Input: part model. Units: mm. Frame: model coordinates. Face numbers are marked on the shaded views. A direction names the side the tool comes from. Give positions to 0.01 mm unless a question says otherwise; leave off trailing zeros. Write each loop counter-clockwise with the first axis right and the second up, starting at its lowest first coordinate (ties: lowest second). Pieces come first, ordered by that corner, then holes. Notation, with made-up numbers: (-25, 60) - (27, 60) arc R31 cw to (27, 90) - close; hole circle Ø5 at (53.5, -8). An arc over 180 degrees is marked (long way). Answer as a JSON object with one key per item and string values. Group by question number.
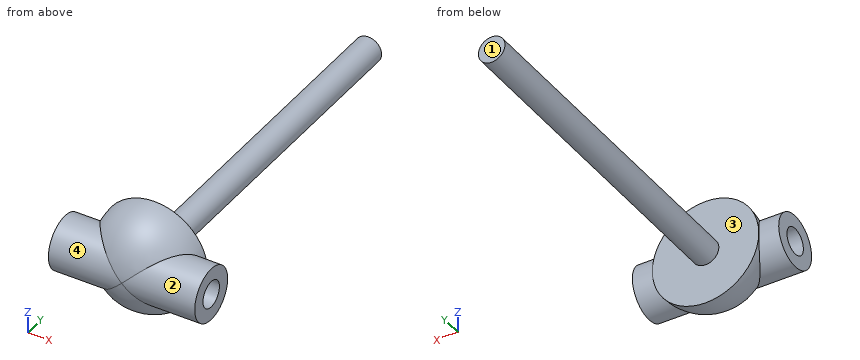
from build123d import *

# Parameters (mm, degrees)
OBR_T1_ANGLE                     = 180
DODANIE_WYCI_GNI_CIE1_DEPTH      = 27.5
DODANIE_WYCI_GNI_CIE1_DEPTH_BACK = 27.5
SZKIC4_R                         = 10
SZKIC5_R                         = 5
WYTNIJ_WYCI_GNI_CIE1_DEPTH       = 62.846584506
SZKIC6_R                         = 5
DODANIE_WYCI_GNI_CIE2_DEPTH      = 130


with BuildPart() as part:
    # Szkic3 → Obr_t1 (revolve)
    with BuildSketch(Plane(origin=(0, 0, 0), x_dir=(1, 0, 0), z_dir=(0, 1, 0))):
        with BuildLine():
            Line((0, 20), (0, -20))
            ThreePointArc((0, -20), (20, 0), (0, 20))
        make_face()
    revolve(axis=Axis((0, 0, -20), (0, 0, -1)), revolution_arc=OBR_T1_ANGLE)

    # Szkic4 → Dodanie-wyci_gni_cie1 (add, two sides: drawn at the far end of the back side and taken through both)
    with BuildSketch(Plane(origin=(0, 0, 0), x_dir=(0, 0, -1), z_dir=(1, 0, 0)).offset(-DODANIE_WYCI_GNI_CIE1_DEPTH_BACK)):
        with Locations((0, -10)):
            Circle(SZKIC4_R)
    extrude(amount=DODANIE_WYCI_GNI_CIE1_DEPTH + DODANIE_WYCI_GNI_CIE1_DEPTH_BACK)

    # Szkic5 → Wytnij-wyci_gni_cie1 (cut, through all)
    with BuildSketch(Plane(origin=(27.5, 0, 0), x_dir=(0, 0, -1), z_dir=(1, 0, 0))):
        with Locations((0, -10)):
            Circle(SZKIC5_R)
    extrude(amount=-WYTNIJ_WYCI_GNI_CIE1_DEPTH, mode=Mode.SUBTRACT)

    # Szkic6 → Dodanie-wyci_gni_cie2 (add)
    with BuildSketch(Plane(origin=(0, 0, 0), x_dir=(1, 0, 0), z_dir=(0, 1, 0))):
        with Locations(Location((0, 0, 0), (0, 0, 180))):
            Circle(SZKIC6_R)
    extrude(amount=DODANIE_WYCI_GNI_CIE2_DEPTH)


solid = part.part
1) Reachability of the marked faces 1, 2, 3 and 4 from +Z, -Z, +X, -X, +Y, -Y: full face, straight path, thin tool, end or side. Return the list, or none.
2) Pin query (flat end, axial travel): P1, Ø4, axis at x = 14, z = 7.5, coming from the +Y side; P2, Ø2, axis at y = 44, z = 1, coming from the +X side; P3, Ø12, axis at x = -3, y = 111, coming from the +Z side. Return the tip coordinate at first contact, or that it passes through.
3) Cut plane D-D on y = 24.5. Return the cut outline in (x, z).
4) Cut plane B-B on y = -10. Return the cut outline in (x, z), and give its area (3 significant figures).
5) Line query: line 1 along Y through (x, z) = (7, 0); line 2 along Y through (x, z) = (3.5, 0); line 3 along Z through (x, y) = (10, -8). Output: solid intervals per line, ascending. Write a range as from..to.
6) Cut plane A-A on x = 3.5. Return the cut outline in (y, z), and give its area (3 significant figures).
7) Cut plane C-C on z = 7.5. Return the cut outline in (x, y), and give its area (3 significant figures).
Filled in:
{
 "1": {"face 1": "+Z, -Z, +X, -X, +Y", "face 2": "+X", "face 3": "+Y", "face 4": "-X"},
 "2": {"P1": "stops at y = 0", "P2": "stops at x = 5", "P3": "stops at z = 5"},
 "3": {"outline": "circle Ø10 at (0, 0)"},
 "4": {"outline": "(-27.5, -10) - (-14.14, -10) arc R17.32 ccw to (14.14, -10) - (27.5, -10) - (27.5, -5) - (-27.5, -5) - close; (-27.5, 5) - (27.5, 5) - (27.5, 10) - (14.14, 10) arc R17.32 ccw to (-14.14, 10) - (-27.5, 10) - close", "area": "840 mm²"},
 "5": {"line 1": "y = -20..-15, -5..0", "line 2": "y = -20..-15, -5..130", "line 3": "z = -15.36..-4.58, 4.58..15.36"},
 "6": {"outline": "(-19.39, -3.45) arc R19.69 ccw to (0, -19.69) - (0, -3.57) - (130, -3.57) - (130, 3.57) - (0, 3.57) - (0, 19.69) arc R19.69 ccw to (-19.39, 3.45) arc R10 ccw to start; hole circle Ø10 at (-10, 0)", "area": "1,460 mm²"},
 "7": {"outline": "(-27.5, -16.61) - (-8.23, -16.61) arc R18.54 ccw to (8.23, -16.61) - (27.5, -16.61) - (27.5, -3.39) - (18.23, -3.39) arc R18.54 ccw to (18.54, 0) - (-18.54, 0) arc R18.54 ccw to (-18.23, -3.39) - (-27.5, -3.39) - close", "area": "874 mm²"}
}
